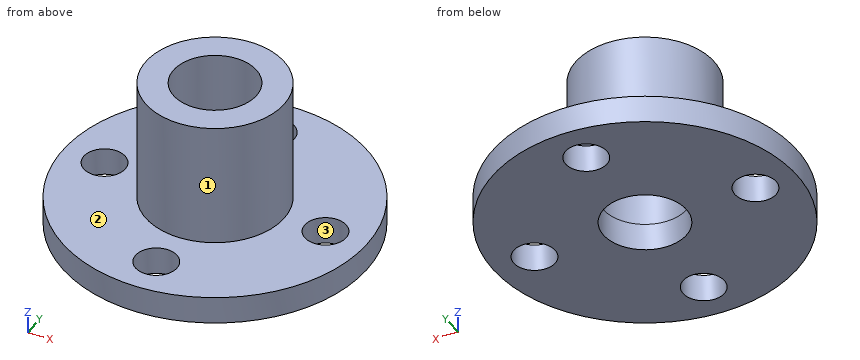
```python
from build123d import *

# Parameters (mm, degrees)
F0_R     = 11
F1_DEPTH = 2
F2_R     = 5
F2_R_2   = 3
F3_DEPTH = 9
F4_R     = 3
F5_DEPTH = 2
F7_D     = 3


with BuildPart() as f1:
    # F0 (on Top) → F1 (new body)
    with BuildSketch(Plane.XY):
        Circle(F0_R)
    extrude(amount=F1_DEPTH)

    # F2 (on face) → F3 (join)
    with BuildSketch(Plane.XY.offset(2)):
        Circle(F2_R)
        Circle(F2_R_2, mode=Mode.SUBTRACT)
    extrude(amount=F3_DEPTH)

    # F4 (on face) → F5 (cut, through all)
    with BuildSketch(Plane.XY.offset(2)):
        Circle(F4_R)
    extrude(amount=-F5_DEPTH, mode=Mode.SUBTRACT)

    # F7 (through all)
    with Locations(Plane.XY.offset(2)):
        with Locations((0, 8), (8, 0), (0, -8), (-8, 0)):
            Hole(F7_D / 2)


solid = f1.part
```
The listing builds one solid part. Answer for the finished solid, in the listing's coordinates (mm). Face numbers are marked on the shaded views. Round coordinates to 2 decimals unless told otherwise and drop trailing zeros. Loops run counter-clockwise (first coordinate to the right, second up) from the corner with the lowest first, then second, coordinate; pieces in that order, holes last.
1) For a pull along X with two mould halves and no side action, classify the marked faces 1, 2 and 3 as released by +X, released by -X, zero draft, split by the parting line, or undercut.
Outcome:
face 1: split by the parting line
face 2: zero draft
face 3: undercut
2) A cutting plane is placed at D-D on x = -0.75. Determine the outline of the cut face in (y, z).
Outcome:
outline: (-10.97, 0) - (-9.3, 0) - (-9.3, 2) - (-10.97, 2) - close; (-6.7, 0) - (-2.9, 0) - (-2.9, 11) - (-4.94, 11) - (-4.94, 2) - (-6.7, 2) - close; (2.9, 0) - (6.7, 0) - (6.7, 2) - (4.94, 2) - (4.94, 11) - (2.9, 11) - close; (9.3, 0) - (10.97, 0) - (10.97, 2) - (9.3, 2) - close
3) A cutting plane is placed at C-C on z = 7.5. Determine the outline of the cut face in (x, y), plus the area to 3 significant figures.
Outcome:
outline: circle Ø10 at (0, 0); hole circle Ø6 at (0, 0)
area: 50.3 mm2
4) Given P1, Ø5, axis at x = 3, y = 8.5, coming from the +Z side; P2, Ø1.5, axis at y = -2.5, z = 8, coming from the +X side; P3, Ø5, axis at x = 0, y = -8, coming from the -Z side; P4, Ø3.5, axis at x = 0, y = 0, coming from the +Z side, each flat-ended and moving along its own axis, determine where each tip first touches the part or whether it passes through.
Outcome:
P1: stops at z = 2
P2: stops at x = 4.68
P3: stops at z = 0
P4: passes through
5) A cutting plane is placed at B-B on x = -8. Determine the outline of the cut face in (y, z).
Outcome:
outline: (-7.55, 0) - (-1.5, 0) - (-1.5, 2) - (-7.55, 2) - close; (1.5, 0) - (7.55, 0) - (7.55, 2) - (1.5, 2) - close
6) A cutting plane is placed at A-A on y = 8.75. Determine the outline of the cut face in (x, z), plus the area to 3 significant figures.
Outcome:
outline: (-6.67, 0) - (-1.3, 0) - (-1.3, 2) - (-6.67, 2) - close; (1.3, 0) - (6.67, 0) - (6.67, 2) - (1.3, 2) - close
area: 21.5 mm2
7) Consider line 1 (Y direction, x = 0, z = 0.55); line 2 (Y direction, x = 0, z = 8.25); line 3 (Z direction, x = -5.5, y = 0.25). Determine where each line is inside the solid, lowest interval first.
Outcome:
line 1: y = -11 to -9.5, -6.5 to -3, 3 to 6.5, 9.5 to 11
line 2: y = -5 to -3, 3 to 5
line 3: z = 0 to 2
